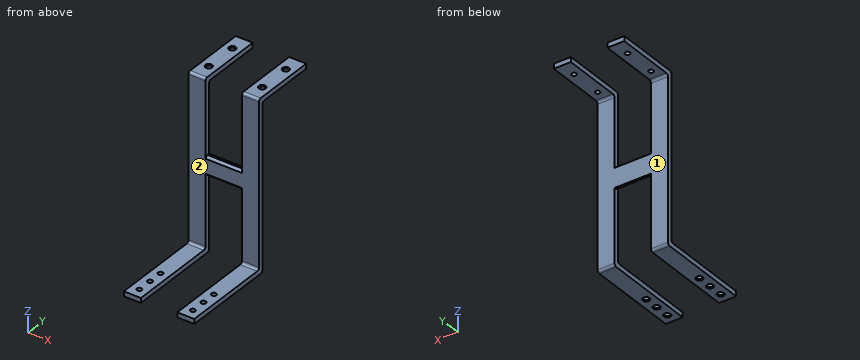
```python
from build123d import *

# Parameters (mm, degrees)
F1_DEPTH = 10
F2_W     = 35
F2_H     = 10
F3_DEPTH = 185
F4_R     = 5
F5_DEPTH = 25
F6_W     = 35
F6_H     = 10
F7_DEPTH = 125
F8_R     = 5
F9_DEPTH = 25
F10_R    = 5
F11_SIZE = 5
F12_SIZE = 2


with BuildPart() as f1:
    # F0 (on Front) → F1 (new body)
    with BuildSketch(Plane.XZ):
        Polygon((-34.9524939805, 272.6582099839), (-69.9524939805, 272.6582099839), (-69.9524939805, -77.3417900161), (-34.9524939805, -77.3417900161), (-34.9524939805, 77.6582099839), (-34.9524939805, 97.6582099839), (-34.9524939805, 117.6582099839), align=None)
        Polygon((40.0475060195, 117.6582099839), (-34.9524939805, 117.6582099839), (-34.9524939805, 97.6582099839), (-34.9524939805, 77.6582099839), (40.0475060195, 77.6582099839), align=None)
        Polygon((40.0475060195, 272.6582099839), (40.0475060195, 117.6582099839), (40.0475060195, 77.6582099839), (40.0475060195, -77.3417900161), (75.0475060195, -77.3417900161), (75.0475060195, 272.6582099839), align=None)
    extrude(amount=F1_DEPTH)

    # F2 (on face) → F3 (join)
    with BuildSketch(Plane.XZ.offset(10)):
        with Locations((-52.4524939805, -72.3417900161)):
            Rectangle(F2_W, F2_H)
        with Locations((57.5475060195, -72.3417900161)):
            Rectangle(F2_W, F2_H)
    extrude(amount=F3_DEPTH)

    # F4 (on face) → F5 (cut)
    with BuildSketch(Plane.XY.offset(-67.3417900161)):
        with Locations((57.5475060195, -114.538833499)):
            Circle(F4_R)
        with Locations((57.5475060195, -144.5381194353)):
            Circle(F4_R)
        with Locations((57.5475060195, -175)):
            Circle(F4_R)
        with Locations((-52.4524939805, -114.538833499)):
            Circle(F4_R)
        with Locations((-52.4524939805, -144.5381194353)):
            Circle(F4_R)
        with Locations((-52.4524939805, -175)):
            Circle(F4_R)
    extrude(amount=-F5_DEPTH, mode=Mode.SUBTRACT)

    # F6 (on face) → F7 (join)
    with BuildSketch(Plane(origin=(0, 0, 0), x_dir=(-1, 0, 0), z_dir=(0, 1, 0))):
        with Locations((-57.5475060195, 267.6582099839)):
            Rectangle(F6_W, F6_H)
        with Locations((52.4524939805, 267.6582099839)):
            Rectangle(F6_W, F6_H)
    extrude(amount=F7_DEPTH)

    # F8 (on face) → F9 (cut)
    with BuildSketch(Plane.XY.offset(272.6582099839)):
        with Locations((-52.4524939805, 23.75)):
            Circle(F8_R)
        with Locations((-52.4524939805, 91.25)):
            Circle(F8_R)
        with Locations((57.5475060195, 91.25)):
            Circle(F8_R)
        with Locations((57.5475060195, 23.75)):
            Circle(F8_R)
    extrude(amount=-F9_DEPTH, mode=Mode.SUBTRACT)

    # F10
    f10_edges = [f1.edges().sort_by_distance(p)[0] for p in [
        (-52.452494, -10, 272.65821),
        (57.547506, -10, 272.65821),
        (-52.452494, -10, -67.34179),
        (57.547506, -10, -67.34179),
        (-52.452494, 0, -77.34179),
        (57.547506, 0, -77.34179),
        (-52.452494, 0, 262.65821),
        (57.547506, 0, 262.65821),
    ]]
    fillet(f10_edges, radius=F10_R)

    # F11
    f11_edges = [f1.edges().sort_by_distance(p)[0] for p in [
        (2.547506, -10, 77.65821),
        (2.547506, -10, 117.65821),
    ]]
    chamfer(f11_edges, length=F11_SIZE)

    # F12
    f12_edges = [f1.edges().sort_by_distance(p)[0] for p in [
        (52.547506, 23.75, 272.65821),
        (52.547506, 91.25, 272.65821),
        (-57.452494, 23.75, 272.65821),
        (-57.452494, 91.25, 272.65821),
        (-57.452494, -175, -77.34179),
        (-57.452494, -144.538119, -77.34179),
        (-57.452494, -114.538833, -77.34179),
        (52.547506, -114.538833, -77.34179),
        (52.547506, -144.538119, -77.34179),
        (52.547506, -175, -77.34179),
    ]]
    chamfer(f12_edges, length=F12_SIZE)


solid = f1.part
```
Model file for the job. Use its own axes, mm. Face numbers are marked on the shaded views. A direction names the side the tool comes from. Round coordinates to 2 decimals unless told otherwise and drop trailing zeros. Order: outer loops, then holes, each group sorted by start corner. A loop starts at its lowest first (then second) coordinate and runs counter-clockwise, first axis right, second up. Notation, with made-up numbers: (22, 27.25) -> (50, 27.25) arc R13 ccw to (50, 48.25) -> close; hole circle Ø10 at (38, -26). An arc over 180 degrees is marked (long way). Use one line per item in the form item = value.
Item 1: Cut at B-B, the plane z = 43. Write the cut outline in (x, y), and give its area (3 significant figures).
Returned:
outline = (-69.95, -10) -> (-34.95, -10) -> (-34.95, 0) -> (-69.95, 0) -> close; (40.05, -10) -> (75.05, -10) -> (75.05, 0) -> (40.05, 0) -> close
area = 700 mm^2
Item 2: Tool access for the marked faces 1 and 2: list every direction of +Z, -Z, +X, -X, +Y, -Y with a clear straight run to the whole face (end or side of a thin tool).
Returned:
face_1 = -Z, +X, -X, +Y
face_2 = +Z, +X, -X, -Y
Item 3: Flat gauge pins, fed straight in: pin 1 Ø10 at (x, z) = (-54, -28.5) entering from -Y; pin 2 Ø16 at (x, y) = (57.55, 91.25) entering from -Z; pin 3 Ø10.5 at (x, y) = (65.5, -131.5) entering from +Z; pin 4 Ø8 at (x, y) = (-52.45, 23.75) entering from +Z. Where does each tip first touch, or does it go through?
Returned:
pin_1 = -10
pin_2 = 262.66
pin_3 = -67.34
pin_4 = through
Item 4: Cut at C-C, the plane y = -175. Write the cut outline in (x, z).
Returned:
outline = (-69.95, -77.34) -> (-59.45, -77.34) -> (-57.45, -75.34) -> (-57.45, -67.34) -> (-69.95, -67.34) -> close; (-47.45, -75.34) -> (-45.45, -77.34) -> (-34.95, -77.34) -> (-34.95, -67.34) -> (-47.45, -67.34) -> close; (40.05, -77.34) -> (50.55, -77.34) -> (52.55, -75.34) -> (52.55, -67.34) -> (40.05, -67.34) -> close; (62.55, -75.34) -> (64.55, -77.34) -> (75.05, -77.34) -> (75.05, -67.34) -> (62.55, -67.34) -> close
Item 5: Cut at A-A, the plane y = 77. Write the cut outline in (x, z).
Returned:
outline = (-69.95, 262.66) -> (-34.95, 262.66) -> (-34.95, 272.66) -> (-69.95, 272.66) -> close; (40.05, 262.66) -> (75.05, 262.66) -> (75.05, 272.66) -> (40.05, 272.66) -> close
Item 6: Drill centre lines: line 1 (X direction, y = 23, z = 268); line 2 (Z direction, x = -63, y = 68); line 3 (Y direction, x = -57, z = -55). Where is each one in solid material? Low to high.
Returned:
line_1 = -69.95 to -57.4, -47.51 to -34.95, 40.05 to 52.6, 62.49 to 75.05
line_2 = 262.66 to 272.66
line_3 = -10 to 0
Item 7: Cut at D-D, the plane x = 27. Write the cut outline in (y, z).
Returned:
outline = (-10, 82.66) -> (-5, 77.66) -> (0, 77.66) -> (0, 117.66) -> (-5, 117.66) -> (-10, 112.66) -> close
